```python
from build123d import *

# Parameters (mm, degrees)
F0_W     = 350
F0_H     = 150
F0_R     = 55
F0_R_2   = 18
F1_DEPTH = 15
F2_R     = 3
F3_ANGLE = 180
F4_R     = 64.95
F5_DEPTH = 5


with BuildPart() as f1:
    # F0 (on Front) → F1 (new body)
    with BuildSketch(Plane.XZ):
        with Locations((2.768559, 0)):
            Rectangle(F0_W, F0_H)
        with Locations((-62.231441, 0)):
            Circle(F0_R, mode=Mode.SUBTRACT)
        with Locations((-139.231441, 42)):
            Circle(F0_R_2, mode=Mode.SUBTRACT)
        with Locations((67.768559, 0)):
            Circle(F0_R, mode=Mode.SUBTRACT)
        with Locations((144.768559, 42)):
            Circle(F0_R_2, mode=Mode.SUBTRACT)
    extrude(amount=F1_DEPTH)

    # F2
    f2_edges = [f1.edges().sort_by_distance(p)[0] for p in [
        (-117.231441, 0, 0),
        (12.768559, 0, 0),
    ]]
    fillet(f2_edges, radius=F2_R)


with BuildPart() as f1_1:
    # F3: moved
    add(f1.part.rotate(Axis((-172.231441, -15, 0), (0, 0, 1)), F3_ANGLE))

    # F4 (on face) → F5 (cut)
    with BuildSketch(Plane(origin=(0, -15, 0), x_dir=(-1, 0, 0), z_dir=(0, 1, 0))):
        with Locations((282.231441, 0)):
            Circle(F4_R)
        with Locations((412.231441, 0)):
            Circle(F4_R)
    extrude(amount=-F5_DEPTH, mode=Mode.SUBTRACT)


solid = f1_1.part
```
CAD build for the part. Positions are in the model's coordinates, mm. A direction names the side the tool comes from. Give positions to 0.01 mm unless a question says otherwise; leave off trailing zeros. Order: outer loops, then holes, each group sorted by start corner. A loop starts at its lowest first (then second) coordinate and runs counter-clockwise, first axis right, second up. Notation, with made-up numbers: M -24.5,63 L -16.5,63 A23 cw -16.5,99 Z; hole C -31,89.25 d3. An arc over 180 degrees is marked long. Put each result on its own line as item: value. Start each with the question number.
(1) Drill centre lines: line 1 along X through (y, z) = (-23, 0); line 2 along X through (y, z) = (-16.5, -37); line 3 along Z through (x, y) = (-204, -28.5). Where is each one in solid material? Low to high.
(2) Flat gauge pin, fed straight in: pin 1 Ø21.5 at (x, z) = (-205.23, 42) entering from +Y (3 decimals). Where does the tip first touch, or does it go through?
(3) Which spindle directions (+Z, -Z, +X, -X, +Y, -Y) get a long thin tool onto all of the face, cutting with end or side? Do faces 1 (the flat face through (-229, -20, 15)), 2 (the flat face through (-345, -15, 18)). Say none if no direction does.
(4) Saw through at A-A, the plane y = -24.5. Write the cut outline in (x, z).
(5) Saw through at D-D, the plane z = 42. Give the number of separate pieces and of enclosed holes in the cut face, then the cut area to 3 significant figures.
(6) Mould opens along Z. For faces 3 (the flat face through (-345, -23, 75)), 4 (the cylindrical face through (-307.6, -23.5, -48.8)), 5 (the flat face through (-172.231, -23, -1)), 6 (the flat face through (-345, -23, -75)) say: +Z half, -Z half, draft (parallel to the pull), parting line (faces both ways), or undercut.
(7) Saw through at C-C, the plane x = -213.5. Write the cut outline in (y, z), then the cut area to 3 significant figures.
(8) Saw through at B-B, the plane z = 0. Write the cut outline in (x, y).
Check result:
1. line 1: x = -522.23 to -467.23, -357.23 to -337.23, -227.23 to -172.23
1. line 2: x = -522.23 to -465.61, -358.85 to -335.61, -228.85 to -172.23
1. line 3: z = -75 to 24.04, 59.96 to 75
2. pin 1: passes through
3. face 1: +Y
3. face 2: +Z, -Z, +X, -X, +Y
4. outline: M -522.23,-75 L -172.23,-75 L -172.23,75 L -522.23,75 Z; hole C -489.23,42 d36; hole C -412.23,0 d110; hole C -282.23,0 d110; hole C -205.23,42 d36
5. separate pieces: 5
5. enclosed holes: 0
5. area: 1,750 mm2
6. face 3: +Z half
6. face 4: undercut
6. face 5: draft
6. face 6: -Z half
7. outline: M -30,-75 L -15,-75 L -15,26.01 L -30,26.01 Z; M -30,57.99 L -15,57.99 L -15,75 L -30,75 Z
7. area: 1,770 mm2
8. outline: M -522.23,-30 L -470.23,-30 A3 ccw -467.23,-27 L -467.23,-20 L -477.18,-20 L -477.18,-15 L -522.23,-15 Z; M -357.23,-27 A3 ccw -354.23,-30 L -340.23,-30 A3 ccw -337.23,-27 L -337.23,-20 L -347.18,-20 L -347.18,-15 L -347.28,-15 L -347.28,-20 L -357.23,-20 Z; M -227.23,-27 A3 ccw -224.23,-30 L -172.23,-30 L -172.23,-15 L -217.28,-15 L -217.28,-20 L -227.23,-20 Z
